Read the model definition and answer for the solid it produces. Units are mm, in the model's axes. Coordinates: 2 decimals unless noted, no trailing zeros. Write each loop counter-clockwise with the first axis right and the second up, starting at its lowest first coordinate (ties: lowest second). Pieces come first, ordered by that corner, then holes. Notation, with made-up numbers: (-28.75, -17) - (-3.75, -17) arc R12 ccw to (-3.75, -12) - close; hole circle Ø4 at (-5.75, 36.5). An arc over 180 degrees is marked (long way). Use a Markdown table: item, result.
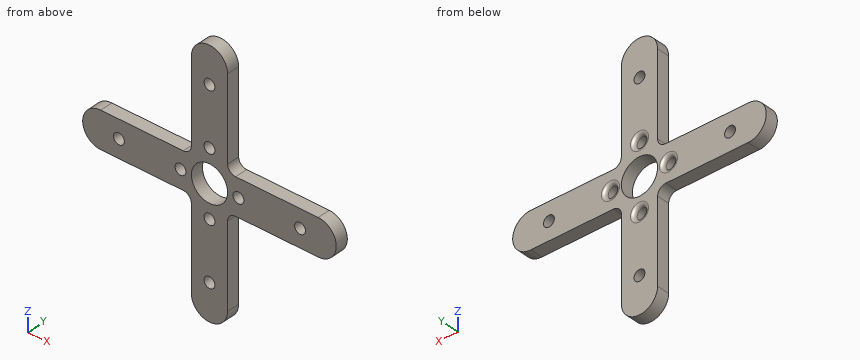
from build123d import *

# Parameters (mm, degrees)
CROQUIS1_R              = 1.5
CROQUIS1_R_2            = 5
SALIENTE_EXTRUIR2_DEPTH = 3.5
REDONDEO9_R             = 1
REDONDEO10_R            = 1
REDONDEO11_R            = 1
REDONDEO12_R            = 1


with BuildPart() as part:
    # Croquis1 → Saliente-Extruir2 (new body)
    with BuildSketch(Plane(origin=(0, 0, 0), x_dir=(1, 0, 0), z_dir=(0, 1, 0))):
        with BuildLine():
            Line((1.47572532, 11.484579709), (1.47572532, 3.695762793))
            ThreePointArc((1.47572532, 3.695762793), (0.818994747, 2.110274939), (-0.766493108, 1.453544366))
            Line((-0.766493108, 1.453544366), (-23.52427468, 1.453544366))
            ThreePointArc((-23.52427468, 1.453544366), (-28.52427468, -3.546455634), (-23.52427468, -8.546455634))
            Line((-23.52427468, -8.546455634), (-0.766493108, -8.546455634))
            ThreePointArc((-0.766493108, -8.546455634), (0.818994747, -9.203186206), (1.47572532, -10.788674061))
            Line((1.47572532, -10.788674061), (1.47572532, -18.577490976))
            Line((1.47572532, -18.577490976), (1.47572532, -33.546455634))
            ThreePointArc((1.47572532, -33.546455634), (6.47572532, -38.546455634), (11.47572532, -33.546455634))
            Line((11.47572532, -33.546455634), (11.47572532, -10.788674061))
            Line((11.47572532, -10.788674061), (11.47572532, -10.748363891))
            ThreePointArc((11.47572532, -10.748363891), (12.133603326, -9.190173106), (13.697697252, -8.546455634))
            Line((13.697697252, -8.546455634), (36.47572532, -8.546455634))
            ThreePointArc((36.47572532, -8.546455634), (41.47572532, -3.546455634), (36.47572532, 1.453544366))
            Line((36.47572532, 1.453544366), (13.697697252, 1.453544366))
            ThreePointArc((13.697697252, 1.453544366), (12.133603326, 2.097261838), (11.47572532, 3.655452623))
            Line((11.47572532, 3.655452623), (11.47572532, 3.695762793))
            Line((11.47572532, 3.695762793), (11.47572532, 26.453544366))
            ThreePointArc((11.47572532, 26.453544366), (6.47572532, 31.453544366), (1.47572532, 26.453544366))
            Line((1.47572532, 26.453544366), (1.47572532, 11.484579709))
        make_face()
        with Locations(Location((-1.52427468, -3.546455634, 0), (0, 0, 270))):
            Circle(CROQUIS1_R, mode=Mode.SUBTRACT)
        with Locations(Location((6.47572532, -28.546455634, 0), (0, 0, 270))):
            Circle(CROQUIS1_R, mode=Mode.SUBTRACT)
        with Locations(Location((6.47572532, -12.546455634, 0), (0, 0, 270))):
            Circle(CROQUIS1_R, mode=Mode.SUBTRACT)
        with Locations(Location((-18.52427468, -3.546455634, 0), (0, 0, 270))):
            Circle(CROQUIS1_R, mode=Mode.SUBTRACT)
        with Locations(Location((6.47572532, -3.546455634, 0), (0, 0, 270))):
            Circle(CROQUIS1_R_2, mode=Mode.SUBTRACT)
        with Locations(Location((14.47572532, -3.546455634, 0), (0, 0, 270))):
            Circle(CROQUIS1_R, mode=Mode.SUBTRACT)
        with Locations(Location((6.47572532, 5.453544366, 0), (0, 0, 270))):
            Circle(CROQUIS1_R, mode=Mode.SUBTRACT)
        with Locations(Location((31.47572532, -3.546455634, 0), (0, 0, 270))):
            Circle(CROQUIS1_R, mode=Mode.SUBTRACT)
        with Locations(Location((6.47572532, 21.453544366, 0), (0, 0, 270))):
            Circle(CROQUIS1_R, mode=Mode.SUBTRACT)
    extrude(amount=SALIENTE_EXTRUIR2_DEPTH)

    # Redondeo9
    redondeo9_edges = [part.edges().sort_by_distance(p)[0] for p in [
        (6.47572532, 3.5, -6.953544366),
    ]]
    fillet(redondeo9_edges, radius=REDONDEO9_R)

    # Redondeo10
    redondeo10_edges = [part.edges().sort_by_distance(p)[0] for p in [
        (14.47572532, 3.5, 2.046455634),
    ]]
    fillet(redondeo10_edges, radius=REDONDEO10_R)

    # Redondeo11
    redondeo11_edges = [part.edges().sort_by_distance(p)[0] for p in [
        (6.47572532, 3.5, 11.046455634),
    ]]
    fillet(redondeo11_edges, radius=REDONDEO11_R)

    # Redondeo12
    redondeo12_edges = [part.edges().sort_by_distance(p)[0] for p in [
        (-1.52427468, 3.5, 2.046455634),
    ]]
    fillet(redondeo12_edges, radius=REDONDEO12_R)


solid = part.part
(1) Straight lines are drawn through the part: L1, parallel to Z at x = 7, y = 2.75; L2, parallel to X at y = 0.9, z = 3; L3, parallel to Z at x = 36.5, y = 0.4. For each, find the intervals that lie inside material, in ascending order.
Report:
| item | result |
|---|---|
| L1 | z = -31.43 to -22.86, -20.05 to -6.89, -4.01 to -1.43, 8.52 to 11.11, 13.99 to 27.14, 29.95 to 38.52 |
| L2 | x = -28.49 to -19.92, -17.13 to -2.92, -0.13 to 1.51, 11.45 to 13.08, 15.87 to 30.08, 32.87 to 41.45 |
| L3 | z = -1.45 to 8.55 |
(2) A cutting plane is placed at C-C, the plane x = -6.5. Write down the section's boundary in (y, z).
Report:
| item | result |
|---|---|
| outline | (0, -1.45) - (3.5, -1.45) - (3.5, 8.55) - (0, 8.55) - close |
(3) A cutting plane is placed at D-D, the plane z = 19. Write down the section's boundary in (x, y), and give its area (3 significant figures).
Report:
| item | result |
|---|---|
| outline | (1.48, 0) - (11.48, 0) - (11.48, 3.5) - (1.48, 3.5) - close |
| area | 35.0 mm² |
(4) Each of these flat-tipped pins is pushed along its axis until it touches: P1, Ø1.5, axis at x = -10.5, y = 1, coming from the -Z side; P2, Ø1.8, axis at y = 2.5, z = -16.5, coming from the +X side; P3, Ø1, axis at x = 30.5, y = 1, coming from the +Z side. Where does it stop, or does it pass through?
Report:
| item | result |
|---|---|
| P1 | stops at z = -1.45 |
| P2 | stops at x = 11.48 |
| P3 | stops at z = 8.55 |
(5) A cutting plane is placed at B-B, the plane y = 0.8. Count the separate pieces of the cut face and the enclosed holes in it, and give its area (3 significant figures).
Report:
| item | result |
|---|---|
| separate pieces | 1 |
| enclosed holes | 9 |
| area | 1,130 mm² |
(6) A cutting plane is placed at A-A, the plane z = -21. Write down the section's boundary in (x, y).
Report:
| item | result |
|---|---|
| outline | (1.48, 0) - (5.05, 0) - (5.05, 3.5) - (1.48, 3.5) - close; (7.91, 0) - (11.48, 0) - (11.48, 3.5) - (7.91, 3.5) - close |
